Build history of the part. All positions in model axes, mm. Round coordinates to 2 decimals unless told otherwise and drop trailing zeros. Write each loop counter-clockwise with the first axis right and the second up, starting at its lowest first coordinate (ties: lowest second). Pieces come first, ordered by that corner, then holes. Notation, with made-up numbers: M 22,17.25 L 30,17.25 A15 cw 30,38.25 Z; hole C 0,-23.75 d1. An arc over 180 degrees is marked long. Use a Markdown table: item, result.
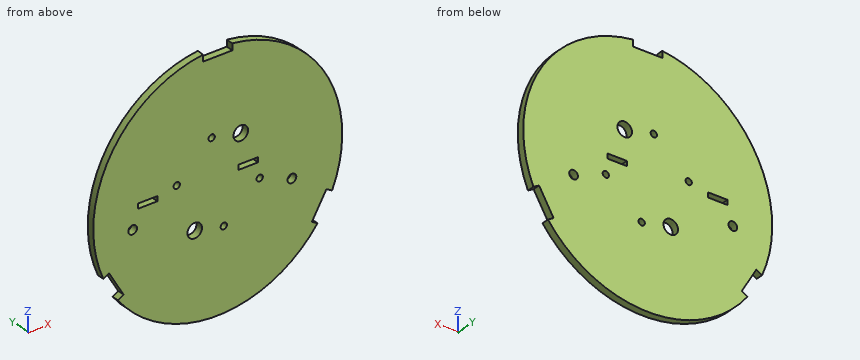
Autodesk Inventor part; units mm, degrees
ref_plane "YZ Plane" through (0, 0, 0) normal (1, 0, 0) x (0, 1, 0)
ref_plane "XZ Plane" through (0, 0, 0) normal (0, 1, 0) x (-1, 0, 0)
ref_plane "XY Plane" through (0, 0, 0) normal (0, 0, 1) x (1, 0, 0)
sketch "Sketch9" plane through (0, 3, 0) normal (0, 1, 0) x (1, 0, 0)
  line L0 (10.4056, -28.6) -> (-19.5944, -28.6)
  line L1 (-19.5944, -28.6) -> (-19.5944, -24.6)
  line L2 (-19.5944, -24.6) -> (10.4056, -24.6)
  line L3 (10.4056, -24.6) -> (10.4056, -28.6)
  point P0 (0, 0)
sketch "Sketch1" plane through (0, 0, 0) normal (0, 1, 0) x (-1, 0, 0)
  circle A0 centre (0, 0) radius 51.35
  dimension "d0" = 102.7
extrude "Plate1" add sketch "Sketch1" along normal blind 3
sketch "Sketch2" plane through (0, 0, 0) normal (0, 1, 0) x (-1, 0, 0)
  line L0 (6, 48.2983) -> (-6, 48.2983)
  line L1 (-6, 48.2983) -> (-6, 53.6983)
  line L2 (-6, 53.6983) -> (6, 53.6983)
  line L3 (6, 53.6983) -> (6, 48.2983)
  line L4 (6, 48.2983) -> (-6, 48.2983)
  line L5 (-6, 48.2983) -> (-6, 50.9983)
  line L6 (-6, 50.9983) -> (6, 50.9983)
  line L7 (6, 50.9983) -> (6, 48.2983)
  circle A0 centre (0, 0) radius 51.35
  point P0 (0, 48.2983)
  point P1 (0, 48.2983)
  dimension "d2" = 2.7
  dimension "d3" = 12
extrude "Cut1" cut sketch "Sketch2" along normal through all contours L0 L1 L6 L3 | A0 L1 L2 L3 | L6 A0
pattern_circular "Circular Pattern1" count 3 over 360 about axis through (0, -10, 0) along (0, 1, 0) of "Cut1"
sketch "Sketch3" plane through (0, 0, 0) normal (0, 1, 0) x (-1, 0, 0)
  point P0 (0, 0)
  point P1 (35.1, -5.8)
  point P2 (-30.6, -9.7)
  dimension "d9" = 5.8
  dimension "d10" = 35.1
  dimension "d11" = 9.7
  dimension "d12" = 30.6
hole "Hole1" at (-35.1, 0, -5.8) at (30.6, 0, -9.7) direction (0, 1, 0) diameter 3.6 end through all
sketch "Sketch4" plane through (0, 3, 0) normal (0, 1, 0) x (1, 0, 0)
  point P0 (0, 0)
  point P1 (-16.9, -4.7)
  point P2 (17.3, 4.8)
  dimension "d20" = 4.7
  dimension "d21" = 16.9
  dimension "d22" = 17.3
  dimension "d23" = 4.8
hole "Hole2" at (-16.9, 3, 4.7) at (17.3, 3, -4.8) direction (0, -1, 0) diameter 2.6 end through all
sketch "Sketch5" plane through (0, 3, 0) normal (0, 1, 0) x (1, 0, 0)
  point P0 (0, 0)
  point P1 (-9.5, 15.3)
  point P2 (9.5, -15.3)
  dimension "d31" = 9.5
  dimension "d32" = 15.3
  dimension "d33" = 9.5
  dimension "d34" = 15.3
hole "Hole3" at (-9.5, 3, -15.3) at (9.5, 3, 15.3) direction (0, -1, 0) diameter 6 end through all
sketch "Sketch6" plane through (0, 3, 0) normal (0, 1, 0) x (1, 0, 0)
  line L0 (-32.9, -1.5) -> (-24.9, -1.5)
  line L1 (-24.9, -1.5) -> (-24.9, -3.5)
  line L2 (-24.9, -3.5) -> (-32.9, -3.5)
  line L3 (-32.9, -3.5) -> (-32.9, -1.5)
  line L4 (8.6, -1.5) -> (16.6, -1.5)
  line L5 (16.6, -1.5) -> (16.6, -3.5)
  line L6 (16.6, -3.5) -> (8.6, -3.5)
  line L7 (8.6, -3.5) -> (8.6, -1.5)
  line L8 (-19.5944, -24.6) -> (10.4056, -24.6)
  line L9 (10.4056, -24.6) -> (10.4056, -28.6)
  line L10 (10.4056, -28.6) -> (-19.5944, -28.6)
  line L11 (-19.5944, -28.6) -> (-19.5944, -24.6)
  point P0 (0, 0)
  dimension "d42" = 8
  dimension "d43" = 8
  dimension "d44" = 33.5
  dimension "d45" = 24.9
  dimension "d46" = 2
  dimension "d47" = 1.5
  dimension "d48" = 21.1
  dimension "d49" = 30
  dimension "d50" = 4
extrude "Cut2" cut sketch "Sketch6" against normal blind 3
sketch "Sketch7" plane through (0, 3, 0) normal (0, 1, 0) x (1, 0, 0)
  point P0 (0, 0)
  point P1 (0, 18)
  point P2 (0, -18)
  dimension "d53" = 18
  dimension "d54" = 18
hole "Hole4" [suppressed]
sketch "Sketch8" plane through (0, 3, 0) normal (0, 1, 0) x (1, 0, 0)
  circle A0 centre (0, 0) radius 18
  point P0 (2.5, 17.8255)
  point P1 (-2.5, -17.8255)
  dimension "d62" = 36
  dimension "d63" = 2.5
  dimension "d64" = 2.5
hole "Hole5" at (2.5, 3, -17.8255) at (-2.5, 3, 17.8255) direction (0, -1, 0) diameter 2.6 end through all
sheet face with bend "Face2" sketch "Sketch9" thickness 3 toward (0, -1, 0) bend radius 3
bend "Bend1"
equation "\"d4\" = Thickness"
equation "\"d18\" = Thickness"
equation "\"d29\" = Thickness"
equation "\"d40\" = Thickness"
equation "\"d51\" = Thickness"
equation "\"d60\" = Thickness"
equation "\"d70\" = Thickness"
equation "\"d77\" = Thickness"
equation "\"d72\" = BendRadius"
equation "\"d73\" = BendReliefWidth"
equation "\"d75\" = MinimumRemnant"
equation "\"d74\" = BendReliefDepth"
equation "\"d76\" = BendRadius"
equation "\"BendRadius\" = Thickness"
equation "\"BendReliefWidth\" = Thickness"
equation "\"BendReliefDepth\" = 0.5 * Thickness"
equation "\"CornerReliefSize\" = 4 * Thickness"
equation "\"MinimumRemnant\" = 2 * Thickness"
equation "\"TransitionRadius\" = BendRadius"
equation "\"JacobiRadiusSize\" = BendRadius"
equation "\"GapSize\" = Thickness"
equation "\"d1\" = BendRadius"
properties part number "LUXCAN BASE DE MONTAJE LENTE"
Q1. Drill centre lines: L1, parallel to X at y = 2.85, z = -17; L2, parallel to Z at x = 9.5, y = 1.1; L3, parallel to X at y = 2.3, z = -5.8. Where is each one in solid material? Low to high.
Response values:
| item | result |
|---|---|
| L1 | x = -48.45 to -11.97, -7.03 to 1.5, 3.5 to 48.45 |
| L2 | z = -50.46 to 1.5, 3.5 to 12.3, 18.3 to 50.46 |
| L3 | x = -51.02 to -36.9, -33.3 to 16.47, 18.13 to 51.02 |
Q2. Drop flat-ended pins along their axis: P1, Ø5.5, axis at x = -9.5, z = -15.3, coming from the -Y side; P2, Ø1, axis at y = 1, z = 2.5, coming from the -X side; P3, Ø0.9, axis at x = -30.5, y = 1, coming from the +Z side; P4, Ø1, axis at y = 0.5, z = 5.5, coming from the +X side. Give the stop position or say it passes through.
Response values:
| item | result |
|---|---|
| P1 | passes through |
| P2 | stops at x = -51.31 |
| P3 | stops at z = 41.64 |
| P4 | stops at x = 51.11 |
Q3. Cut at D-D on x = 42.5. Give the cut face in (y, z), and give its area (3 significant figures).
Response values:
| item | result |
|---|---|
| outline | M 0,-22.98 L 3,-22.98 L 3,28.82 L 0,28.82 Z |
| area | 155 mm2 |
Q4. Cut at C-C on x = -29. Give the cut face in (y, z).
Response values:
| item | result |
|---|---|
| outline | M 0,-42.38 L 3,-42.38 L 3,1.5 L 0,1.5 Z; M 0,3.5 L 3,3.5 L 3,42.38 L 0,42.38 Z |
Q5. Cut at B-B on z = -15.3. Give the cut face in (x, y), and give its area (3 significant figures).
Response values:
| item | result |
|---|---|
| outline | M -49.02,0 L -12.5,0 L -12.5,3 L -49.02,3 Z; M -6.5,0 L 49.02,0 L 49.02,3 L -6.5,3 Z |
| area | 276 mm2 |
Q6. Cut at A-A on y = 2.15. Count the separate pieces of the cut face and the enclosed holes in it, and give its area (3 significant figures).
Response values:
| item | result |
|---|---|
| separate pieces | 1 |
| enclosed holes | 10 |
| area | 8,050 mm2 |
